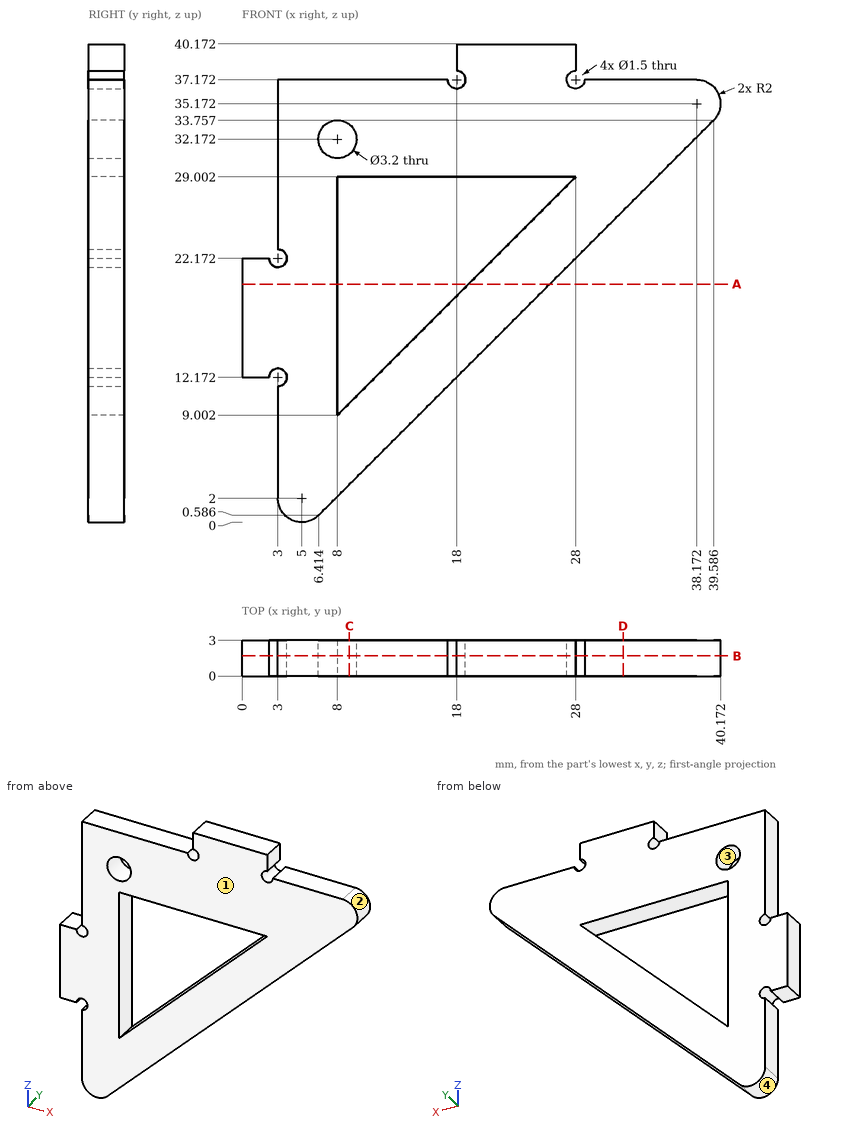
Check sheet for the drawn part. Datum: minimum x, y, z corner. Units: mm. Coordinates: 2 decimals unless noted, no trailing zeros. Write each loop counter-clockwise with the first axis right and the second up, starting at its lowest first coordinate (ties: lowest second). Pieces come first, ordered by that corner, then holes. Notation, with made-up numbers: M -11.75,75.5 L 0.25,75.5 A18 cw 0.25,88.5 Z; hole C 21,27 d6. An arc over 180 degrees is marked long. Use a Markdown table: item, result.
Q1. Thickness scan on line 1 (X direction, y = 0.8, z = 37) (1 decimal); line 2 (X direction, y = 2.65, z = 24); line 3 (X direction, y = 1.8, z = 38.5). Record the ranges inside material, lowest first.
Reply:
| item | result |
|---|---|
| line 1 | x = 3 to 17.3, 18.7 to 27.3, 28.7 to 39 |
| line 2 | x = 3 to 8, 23 to 29.83 |
| line 3 | x = 18 to 28 |
Q2. Sectioned sample at B-B, the plane y = 1.7. Count the separate pieces of the cut face and the enclosed holes in it, plus the area to 3 significant figures.
Reply:
| item | result |
|---|---|
| separate pieces | 1 |
| enclosed holes | 2 |
| area | 637 mm² |
Q3. Sectioned sample at C-C, the plane x = 9. Record the boundary of the cut face in (y, z).
Reply:
| item | result |
|---|---|
| outline | M 0,3.17 L 3,3.17 L 3,10 L 0,10 Z; M 0,29 L 3,29 L 3,30.92 L 0,30.92 Z; M 0,33.42 L 3,33.42 L 3,37.17 L 0,37.17 Z |
Q4. Sectioned sample at D-D, the plane x = 32. Record the boundary of the cut face in (y, z), plus the area to 3 significant figures.
Reply:
| item | result |
|---|---|
| outline | M 0,26.17 L 3,26.17 L 3,37.17 L 0,37.17 Z |
| area | 33.0 mm² |
Q5. Sectioned sample at A-A, the plane z = 20. Record the boundary of the cut face in (x, y).
Reply:
| item | result |
|---|---|
| outline | M 0,0 L 8,0 L 8,3 L 0,3 Z; M 19,0 L 25.83,0 L 25.83,3 L 19,3 Z |
Q6. Go/stop test with flat-tipped pins: P1, Ø0.9, axis at y = 2, z = 7, coming from the -X side; P2, Ø1.5, axis at x = 34.5, y = 1.5, coming from the -Z side; P3, Ø1.5, axis at x = 35.5, y = 0.5, coming from the -Z side. Record where each tip stops, or that it passes through.
Reply:
| item | result |
|---|---|
| P1 | stops at x = 3 |
| P2 | stops at z = 27.92 |
| P3 | stops at z = 28.92 |
Q7. Draft check along Z on the marked faces 1, 2, 3 and 4. Enter one of: +Z half, -Z half, draft (parallel to the pull), parting line (faces both ways), or undercut.
Reply:
| item | result |
|---|---|
| face 1 | draft |
| face 2 | parting line |
| face 3 | undercut |
| face 4 | -Z half |
